Answer from the drawing. Dimensions are ordinates in mm from the lowest x, y and z of the part. Coordinates: 2 decimals unless noted, no trailing zeros. Write each loop counter-clockwise with the first axis right and the second up, starting at its lowest first coordinate (ties: lowest second). Pieces come first, ordered by that corner, then holes. Notation, with made-up numbers: (74.5, 15.5) - (128.5, 15.5) arc R27 ccw to (128.5, 42.5) - close; hole circle Ø1 at (34.25, 60). An arc over 180 degrees is marked (long way). Use one line per item in the form item = value. Start each with the question number.
Item 1: Determine the mould class of the marked faces 1 and 2 for opening direction X: released by +X, released by -X, zero draft, split by the parting line, or undercut.
Item 2: A cutting plane is placed at D-D (x = 57.5). Write down the section's boundary in (y, z), then the cut area to 3 significant figures.
Item 3: Given pin 1 (11.5 mm diameter, centred on x = 94, z = 90, fed in from -Y), flat-ended and moving along its own axis, determine where the tip first touches the part or whether it passes through.
Item 4: A cutting plane is placed at B-B (z = 96). Write down the section's boundary in (x, y), then the cut area to 3 significant figures.
Item 5: Consider probe 1 along Z at (x, y) = (110, 3.75) (3 decimals); probe 2 along Z at (x, y) = (64.5, 5); probe 3 along X at (y, z) = (1.25, 81.5). Determine where each line is inside the solid, lowest interval first.
Item 6: A cutting plane is placed at A-A (x = 34). Write down the section's boundary in (y, z), then the cut area to 3 significant figures.
Item 7: A cutting plane is placed at C-C (y = 4.75). Write down the section's boundary in (x, z) (3 decimals).
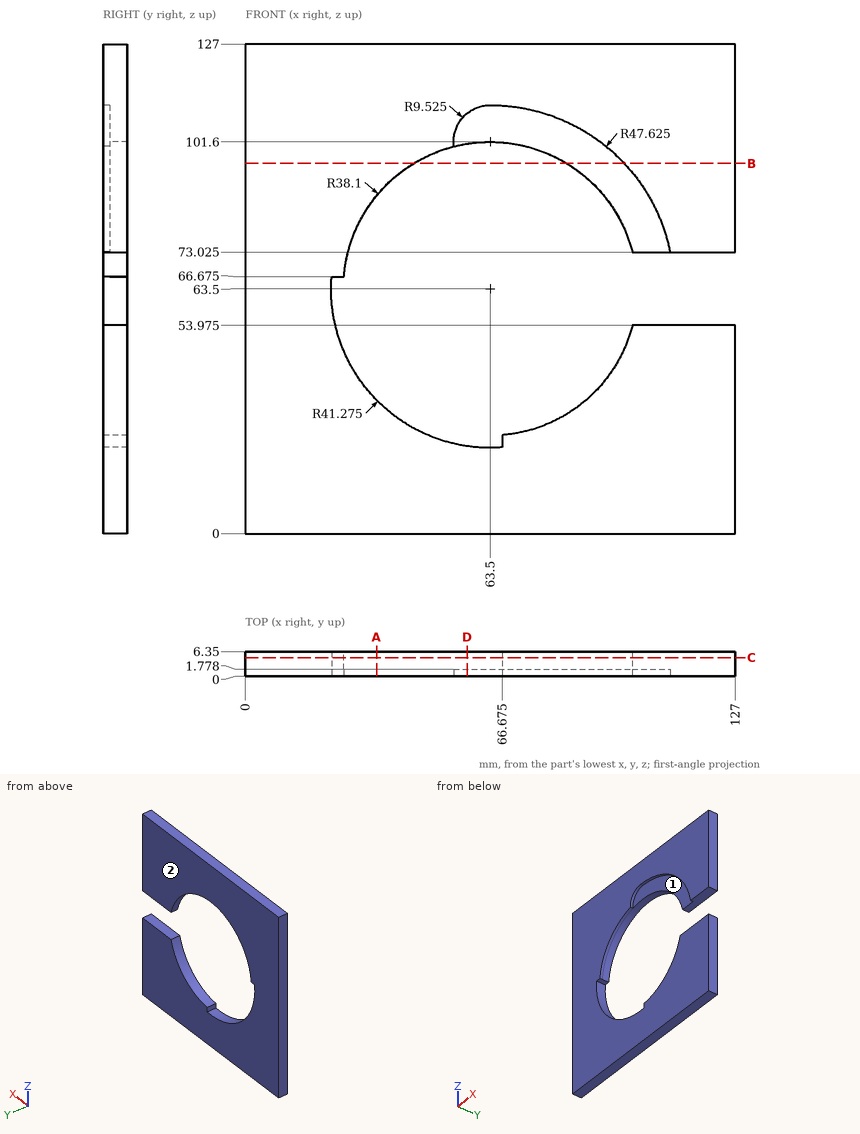
Answer:
q1.face_1 = undercut
q1.face_2 = zero draft
q2.outline = (0, 0) - (6.35, 0) - (6.35, 22.66) - (0, 22.66) - close; (0, 109) - (1.78, 109) - (1.78, 101.12) - (6.35, 101.12) - (6.35, 127) - (0, 127) - close
q2.area = 294 mm²
q3.pin_1 = 1.78
q4.outline = (0, 0) - (43.62, 0) - (43.62, 6.35) - (0, 6.35) - close; (83.38, 1.78) - (98.31, 1.78) - (98.31, 0) - (127, 0) - (127, 6.35) - (83.38, 6.35) - close
q4.area = 527 mm²
q5.probe_1 = 0 to 53.975, 73.025 to 127
q5.probe_2 = 0 to 22.24, 101.59 to 127
q5.probe_3 = 0 to 29.92, 107.59 to 127
q6.outline = (0, 0) - (6.35, 0) - (6.35, 34.63) - (0, 34.63) - close; (0, 87.61) - (6.35, 87.61) - (6.35, 127) - (0, 127) - close
q6.area = 470 mm²
q7.outline = (0, 0) - (127, 0) - (127, 53.975) - (100.39, 53.975) arc R38.1 cw to (66.675, 25.533) - (66.675, 22.347) arc R41.275 cw to (22.347, 66.675) - (25.533, 66.675) arc R38.1 cw to (100.39, 73.025) - (127, 73.025) - (127, 127) - (0, 127) - close
